Autodesk Fusion 360 part; units mm, degrees
sketch "Sketch1" plane through (0, 0, 0) normal (0, 1, 0) x (1, 0, 0)
  line L0 (12, -9) -> (-12, -9)
  line L1 (-12, -9) -> (-12, 9)
  line L2 (-12, 9) -> (12, 9)
  line L3 (12, 9) -> (12, -9)
  line L4 (12, -9) -> (-12, 9) construction
  line L5 (-12, -9) -> (12, 9) construction
  dimension "d1" = 24
  dimension "d2" = 18
extrude "Extrude1" add sketch "Sketch1" along normal blind 7
fillet "Fillet1" radius 2 12 edges at (-12, 3.5, 9) (0, 7, 9) (0, 0, 9) (12, 3.5, 9) (12, 7, 0) (12, 0, 0) (12, 3.5, -9) (0, 7, -9) (0, 0, -9) (-12, 3.5, -9) (-12, 7, 0) (-12, 0, 0)
sketch "Sketch2" plane through (-12, 0, 0) normal (-1, 0, 0) x (0, 0, 1)
  line L0 (-7, 2) -> (7, 2)
  line L1 (7, 2) -> (7, 5)
  line L2 (7, 5) -> (-7, 5)
  line L3 (-7, 5) -> (-7, 2)
  line L4 (-7, 3.5) -> (7, 3.5) construction
  circle A0 centre (0, 3.5) radius 1.5
  circle A1 centre (0, 3.5) radius 1.1
  circle A2 centre (-5.5, 3.5) radius 1.5
  circle A3 centre (5.5, 3.5) radius 1.5
  circle A4 centre (5.5, 3.5) radius 1.1
  circle A5 centre (-5.5, 3.5) radius 1.1
  dimension "d6" = 2.2
extrude "Extrude2" add sketch "Sketch2" along normal blind 4 contours A2 | A0 | A3
sketch "Sketch3" plane through (12, 0, 0) normal (1, 0, 0) x (0, 0, -1)
  line L0 (-7, 2) -> (7, 2)
  line L1 (7, 2) -> (7, 5)
  line L2 (7, 5) -> (-7, 5)
  line L3 (-7, 5) -> (-7, 2)
  line L4 (7, 3.5) -> (-7, 3.5) construction
  line L5 (6.3632, 4.5) -> (1.8632, 4.5)
  line L6 (1.8632, 4.5) -> (1.8632, 2.5)
  line L7 (1.8632, 2.5) -> (6.3632, 2.5)
  line L8 (6.3632, 2.5) -> (6.3632, 4.5)
  line L9 (6.3632, 4.5) -> (1.8632, 2.5) construction
  line L10 (1.8632, 4.5) -> (6.3632, 2.5) construction
  circle A0 centre (-5.5, 3.5) radius 1.5
  circle A1 centre (-5.5, 3.5) radius 1.1
  circle A2 centre (0, 3.5) radius 1.5
  circle A3 centre (0, 3.5) radius 1.1
  point P0 (4.1132, 3.5)
  dimension "d10" = 4.5
  dimension "d11" = 1
  dimension "d12" = 3
  dimension "d13" = 2.2
extrude "Extrude3" add sketch "Sketch3" along normal blind 4 contours A0 | A2 | L5 L6 L7 L8
Input: part model. Units: mm. Frame: model coordinates. A direction names the side the tool comes from. Coordinates: 2 decimals unless noted, no trailing zeros. Order: outer loops, then holes, each group sorted by start corner. A loop starts at its lowest first (then second) coordinate and runs counter-clockwise, first axis right, second up. Notation, with made-up numbers: (15, 32) - (45, 32) arc R9 ccw to (45, 44) - close; hole circle Ø4 at (45.25, 29). An arc over 180 degrees is marked (long way). Put each result on its own line as item: value.
1. Draft query along Z for faces 5 (the face through (14, 2.5, -4)), 6 (the face through (-13.97, 2.57, -4.91)), 7 (the face through (-11.43, 3.52, 8.4)), 8 (the face through (14, 3, -6.363)). Return one class per face: pulls with the +Z half, pulls with the -Z half, needs draft (parallel to the pull), parting line crosses it, or undercut.
Report:
face 5: needs draft
face 6: undercut
face 7: pulls with the +Z half
face 8: pulls with the -Z half
2. Reachability of faces 1 (the face through (14, 4.5, -4)), 2 (the face through (12, 3, 5)), 3 (the face through (12, 4.7, 6.7)), 4 (the face through (14, 4, -1.863)) from +Z, -Z, +X, -X, +Y, -Y: full face, straight path, thin tool, end or side. Return the list, or none.
Report:
face 1: -Z, +X, +Y
face 2: +X
face 3: +Z, +X, +Y
face 4: +X, +Y, -Y
3. Contact query for flat-ended pins moving along their axis: pin 1 Ø1.8 at (y, z) = (3.5, 5.5) entering from +X; pin 2 Ø1.8 at (y, z) = (3.5, 0) entering from -X; pin 3 Ø1 at (x, y) = (13.5, 3.5) entering from +Z. Output: stop coordinate, or through.
Report:
pin 1: stops at x = 12
pin 2: stops at x = -12
pin 3: stops at z = 7
4. Line query: line 1 along Y through (x, z) = (14.55, 0); line 2 along Z through (x, y) = (-14, 4.25); line 3 along X through (y, z) = (2, -2). Output: solid intervals per line, ascending.
Report:
line 1: y = 2 to 2.4, 4.6 to 5
line 2: z = -6.8 to -6.3, -4.7 to -4.2, -1.3 to -0.8, 0.8 to 1.3, 4.2 to 4.7, 6.3 to 6.8
line 3: x = -12 to 12
5. Cut plane A-A on x = 3.5. Return the cut outline in (y, z).
Report:
outline: (0, -7) arc R2 ccw to (2, -9) - (5, -9) arc R2 ccw to (7, -7) - (7, 7) arc R2 ccw to (5, 9) - (2, 9) arc R2 ccw to (0, 7) - close
6. Cut plane B-B on z = 7.75. Return the cut outline in (x, y).
Report:
outline: (-11.85, 2) arc R1.85 ccw to (-10, 0.15) - (10, 0.15) arc R1.85 ccw to (11.85, 2) - (11.85, 5) arc R1.85 ccw to (10, 6.85) - (-10, 6.85) arc R1.85 ccw to (-11.85, 5) - close
